The figure shows three views and two pictorial views of one solid part (mm, origin at its lowest corner). Answer the questions. Coordinates: 2 decimals unless noted, no trailing zeros. Write each loop counter-clockwise with the first axis right and the second up, starting at its lowest first coordinate (ties: lowest second). Pieces come first, ordered by that corner, then holes.
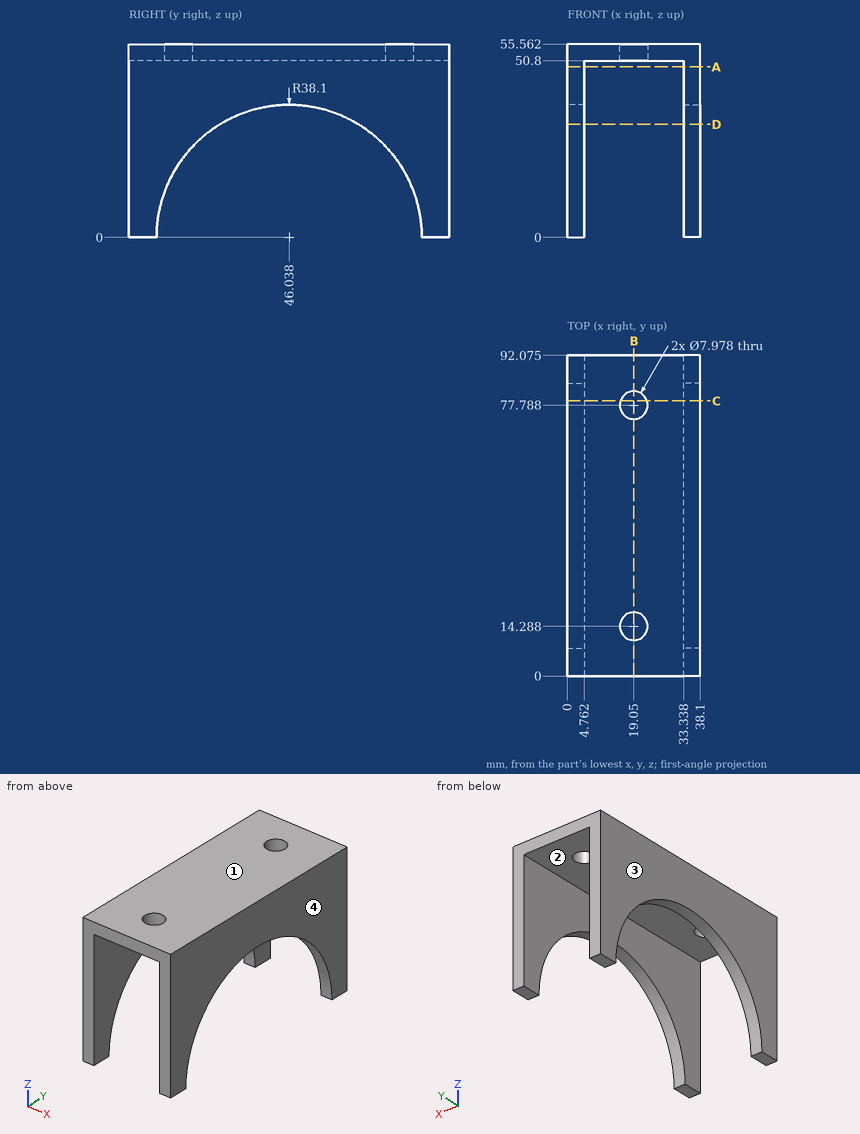
Item 1: The part is cut by section C-C (y = 79). Give the vertices of the cut face in (x, z).
Item 2: The part is cut by section A-A (z = 49). Give the vertices of the cut face in (x, y) (1 decimal).
Item 3: The part is cut by section D-D (z = 32.5). Give the vertices of the cut face in (x, y) (1 decimal), and give its area (3 significant figures).
Item 4: Given pin 1 (5 mm diameter, centred on y = 16.5, z = 43.5, fed in from -X); pin 2 (3 mm diameter, centred on x = 9.5, y = 70, fed in from -Z), each flat-ended and moving along its own axis, determine where each tip first touches the part or whether it passes through.
Item 5: Determine the mould class of the marked faces 1, 2, 3 and 4 for opening direction X: +X half, -X half, draft (parallel to the pull), parting line (faces both ways), or undercut.
Item 6: Find the intervals of material crossed by probe 1 along Y at (x, z) = (19.05, 53.6) (1 decimal); probe 2 along X at (y, z) = (47, 41.5); probe 3 along Z at (x, y) = (28, 70), in increasing order.
Item 7: The part is cut by section B-B (x = 19.05). Give the vertices of the cut face in (y, z) (1 decimal).
Answer:
1. outline: (0, 19.11) - (4.76, 19.11) - (4.76, 50.8) - (15.25, 50.8) - (15.25, 55.56) - (0, 55.56) - close; (22.85, 50.8) - (33.34, 50.8) - (33.34, 19.11) - (38.1, 19.11) - (38.1, 55.56) - (22.85, 55.56) - close
2. outline: (0, 0) - (4.8, 0) - (4.8, 92.1) - (0, 92.1) - close; (33.3, 0) - (38.1, 0) - (38.1, 92.1) - (33.3, 92.1) - close
3. outline: (0, 0) - (4.8, 0) - (4.8, 26.2) - (0, 26.2) - close; (0, 65.9) - (4.8, 65.9) - (4.8, 92.1) - (0, 92.1) - close; (33.3, 0) - (38.1, 0) - (38.1, 26.2) - (33.3, 26.2) - close; (33.3, 65.9) - (38.1, 65.9) - (38.1, 92.1) - (33.3, 92.1) - close
3. area: 498 mm2
4. pin 1: stops at x = 0
4. pin 2: stops at z = 50.8
5. face 1: draft
5. face 2: undercut
5. face 3: -X half
5. face 4: +X half
6. probe 1: y = 0 to 10.3, 18.3 to 73.8, 81.8 to 92.1
6. probe 2: x = 0 to 4.76, 33.34 to 38.1
6. probe 3: z = 50.8 to 55.56
7. outline: (0, 50.8) - (10.3, 50.8) - (10.3, 55.6) - (0, 55.6) - close; (18.3, 50.8) - (73.8, 50.8) - (73.8, 55.6) - (18.3, 55.6) - close; (81.8, 50.8) - (92.1, 50.8) - (92.1, 55.6) - (81.8, 55.6) - close
